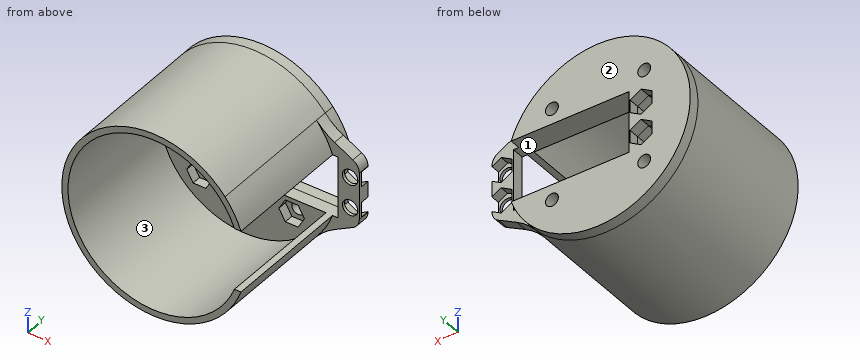
```python
from build123d import *

# Parameters (mm, degrees)
SKETCH_1_R          = 2.5
SKETCH_1_W          = 40
SKETCH_1_H          = 20
EXTRUDE_3_DEPTH     = 4
EXTRUDE_START       = 42
EXTRUDE_16_DEPTH    = 42
CUT_EXTRUDE_1_DEPTH = 3
EXTRUDE_4_DEPTH     = 3.5
CUT_EXTRUDE_2_DEPTH = 3
SKETCH_6_R          = 2.1
CUT_EXTRUDE_3_DEPTH = 66.299310869


with BuildPart() as part:
    # 草图1 → 凸台-拉伸3 (new body)
    with BuildSketch(Plane(origin=(0, 0, 0), x_dir=(1, 0, 0), z_dir=(0, 1, 0))):
        with BuildLine():
            Line((18.956802834, 14.347674144), (24.902068137, 11.134017223))
            ThreePointArc((24.902068137, 11.134017223), (26.435714813, 9.663571926), (27, 7.615191169))
            Line((27, 7.615191169), (27, -7.615191169))
            ThreePointArc((27, -7.615191169), (26.435714813, -9.663571926), (24.902068137, -11.134017223))
            Line((24.902068137, -11.134017223), (18.956802834, -14.347674144))
            ThreePointArc((18.956802834, -14.347674144), (15.787653215, -16.474725649), (13.080286113, -19.165082649))
            ThreePointArc((13.080286113, -19.165082649), (-40, 0), (13.080286113, 19.165082649))
            ThreePointArc((13.080286113, 19.165082649), (15.787653215, 16.474725649), (18.956802834, 14.347674144))
        make_face()
        with Locations(Location((24, 5, 0), (0, 0, 270))):
            Circle(SKETCH_1_R, mode=Mode.SUBTRACT)
        with Locations(Location((24, -5, 0), (0, 0, 270))):
            Circle(SKETCH_1_R, mode=Mode.SUBTRACT)
        with Locations(Location((-24, 5, 0), (0, 0, 270))):
            Circle(SKETCH_1_R, mode=Mode.SUBTRACT)
        with Locations(Location((-24, -5, 0), (0, 0, 270))):
            Circle(SKETCH_1_R, mode=Mode.SUBTRACT)
        Rectangle(SKETCH_1_W, SKETCH_1_H, mode=Mode.SUBTRACT)
    extrude(amount=EXTRUDE_3_DEPTH)

    # 草图10 → 凸台-拉伸16 (add)
    with BuildSketch(Plane.XZ.offset(EXTRUDE_START)):
        with BuildLine():
            Line((16.153393661, 10), (18.284271247, 10))
            ThreePointArc((18.284271247, 10), (16.087911438, 14.812861871), (13.080286113, 19.165082649))
            ThreePointArc((13.080286113, 19.165082649), (-40, 0), (13.080286113, -19.165082649))
            ThreePointArc((13.080286113, -19.165082649), (16.087911438, -14.812861871), (18.284271247, -10))
            Line((18.284271247, -10), (16.153393661, -10))
            ThreePointArc((16.153393661, -10), (-38, 0), (16.153393661, 10))
        make_face()
    extrude(amount=-EXTRUDE_16_DEPTH)

    # 草图2 → 切除-拉伸1 (cut)
    with BuildSketch(Plane(origin=(0, 4, 0), x_dir=(1, 0, 0), z_dir=(0, 1, 0))):
        Polygon((24, 0.843078062), (27.6, 2.921539031), (27.6, 7.078460969), (24, 9.156921938), (20.4, 7.078460969), (20.4, 2.921539031), align=None)
        Polygon((-24, 0.843078062), (-20.4, 2.921539031), (-20.4, 7.078460969), (-24, 9.156921938), (-27.6, 7.078460969), (-27.6, 2.921539031), align=None)
        Polygon((24, -9.156921938), (27.6, -7.078460969), (27.6, -2.921539031), (24, -0.843078062), (20.4, -2.921539031), (20.4, -7.078460969), align=None)
        Polygon((-24, -9.156921938), (-20.4, -7.078460969), (-20.4, -2.921539031), (-24, -0.843078062), (-27.6, -2.921539031), (-27.6, -7.078460969), align=None)
    extrude(amount=-CUT_EXTRUDE_1_DEPTH, mode=Mode.SUBTRACT)

    # 草图3 → 凸台-拉伸4 (add)
    with BuildSketch(Plane(origin=(0, 4, 0), x_dir=(1, 0, 0), z_dir=(0, 1, 0))):
        with BuildLine():
            Line((18.284271247, -10), (-20, -10))
            Line((-20, -10), (-20, 10))
            Line((-20, 10), (18.284271247, 10))
            ThreePointArc((18.284271247, 10), (16.087911438, 14.812861871), (13.080286113, 19.165082649))
            ThreePointArc((13.080286113, 19.165082649), (-40, 0), (13.080286113, -19.165082649))
            ThreePointArc((13.080286113, -19.165082649), (16.087911438, -14.812861871), (18.284271247, -10))
        make_face()
        Polygon((-20.4, -7.078460969), (-24, -9.156921938), (-27.6, -7.078460969), (-27.6, -2.921539031), (-24, -0.843078062), (-20.4, -2.921539031), align=None, mode=Mode.SUBTRACT)
        Polygon((-20.4, 2.921539031), (-24, 0.843078062), (-27.6, 2.921539031), (-27.6, 7.078460969), (-24, 9.156921938), (-20.4, 7.078460969), align=None, mode=Mode.SUBTRACT)
    extrude(amount=EXTRUDE_4_DEPTH)

    # 草图4 → 切除-拉伸2 (cut)
    with BuildSketch(Plane.XZ):
        Polygon((9.156921938, 15), (7.078460969, 18.6), (2.921539031, 18.6), (0.843078062, 15), (2.921539031, 11.4), (7.078460969, 11.4), align=None)
        Polygon((-20.843078062, 15), (-22.921539031, 18.6), (-27.078460969, 18.6), (-29.156921938, 15), (-27.078460969, 11.4), (-22.921539031, 11.4), align=None)
        Polygon((9.156921938, -15), (7.078460969, -11.4), (2.921539031, -11.4), (0.843078062, -15), (2.921539031, -18.6), (7.078460969, -18.6), align=None)
        Polygon((-20.843078062, -15), (-22.921539031, -11.4), (-27.078460969, -11.4), (-29.156921938, -15), (-27.078460969, -18.6), (-22.921539031, -18.6), align=None)
    extrude(amount=-CUT_EXTRUDE_2_DEPTH, mode=Mode.SUBTRACT)

    # 草图6 → 切除-拉伸3 (cut, through all)
    with BuildSketch(Plane.XZ):
        with Locations(Location((-25, 15, 0), (0, 0, 270))):
            Circle(SKETCH_6_R)
        with Locations(Location((5, 15, 0), (0, 0, 270))):
            Circle(SKETCH_6_R)
        with Locations(Location((5, -15, 0), (0, 0, 270))):
            Circle(SKETCH_6_R)
        with Locations(Location((-25, -15, 0), (0, 0, 270))):
            Circle(SKETCH_6_R)
    extrude(amount=-CUT_EXTRUDE_3_DEPTH, mode=Mode.SUBTRACT)


solid = part.part
```
Read the model definition and answer for the solid it produces. Units are mm, in the model's axes. Face numbers are marked on the shaded views. A direction names the side the tool comes from. Give positions to 0.01 mm unless a question says otherwise; leave off trailing zeros. Order: outer loops, then holes, each group sorted by start corner. A loop starts at its lowest first (then second) coordinate and runs counter-clockwise, first axis right, second up. Notation, with made-up numbers: (59.5, 71) -> (90.5, 71) arc R31 ccw to (90.5, 98) -> close; hole circle Ø5 at (5, 54.5). An arc over 180 degrees is marked (long way). One line per item, written item: value. Start each with the question number.
(1) The part is cut by section A-A (z = 0). Determine the outline of the cut face in (x, y).
(2) Straight lines are drawn through the part: L1, parallel to Z at x = -24, y = 0.4; L2, parallel to X at y = 6.1, z = -15; L3, parallel to Y at x = -12.5, z = -11. For each, find the intervals that lie inside material, in ascending order.
(3) The part is cut by section B-B (x = -14). Determine the outline of the cut face in (y, z).
(4) The part is cut by section C-C (y = -14.5). Determine the outline of the cut face in (x, z), and give its area (3 significant figures).
(5) The part is cut by section D-D (z = 20). Determine the outline of the cut face in (x, y).
(6) Flat-ended cylindrical pins translate along their axes: P1, Ø1.5, axis at y = -8, z = -17.5, coming from the +X side; P2, Ø3.5, axis at x = -25.5, z = -4.5, coming from the +Y side; P3, Ø10, axis at x = 0, y = -10.5, coming from the +Z side; P4, Ø3.5, axis at x = -25, z = 15, coming from the +Y side. Find the tip coordinate at first contact, or state that the pin passes through.
(7) A tool of negligible diameter and unlimited length cuts with its end or side. For the marked faces 1, 2 and 3, from which of +Z, -Z, +X, -X, +Y, -Y can it reach the whole face along a straight path? Write none if from no direction.
Taken from the geometry:
1. outline: (-40, -42) -> (-38, -42) -> (-38, 0) -> (-20, 0) -> (-20, 7.5) -> (-40, 7.5) -> close; (20, 0) -> (27, 0) -> (27, 4) -> (20, 4) -> close
2. L1: -26.53 to -18.6, -11.4 to -7.5, -2.5 to 2.5, 7.5 to 11.4, 18.6 to 26.53
2. L2: -35.98 to -27.1, -22.9 to 2.9, 7.1 to 15.98
2. L3: 0 to 7.5
3. outline: (-42, -29.73) -> (7.5, -29.73) -> (7.5, -10) -> (0, -10) -> (0, -27.71) -> (-42, -27.71) -> close; (-42, 27.71) -> (0, 27.71) -> (0, 10) -> (7.5, 10) -> (7.5, 29.73) -> (-42, 29.73) -> close
4. outline: (16.15, -10) arc R28 cw (long way) to (16.15, 10) -> (18.28, 10) arc R30 ccw (long way) to (18.28, -10) -> close
4. area: 324 mm^2
5. outline: (-32.36, -42) -> (-29.6, -42) -> (-29.6, 0) -> (9.6, 0) -> (9.6, -42) -> (12.36, -42) -> (12.36, 7.5) -> (-32.36, 7.5) -> close
6. P1: x = 14.89
6. P2: y = 1
6. P3: z = 29.58
6. P4: through
7. face 1: +Y, -Y
7. face 2: +Z, -Z, +X, -X, +Y
7. face 3: -Y
